The model under review builds one solid part; all positions refer to its coordinate system, in mm. A direction names the side the tool comes from. Round coordinates to 2 decimals unless told otherwise and drop trailing zeros. Order: outer loops, then holes, each group sorted by start corner. A loop starts at its lowest first (then second) coordinate and runs counter-clockwise, first axis right, second up. Notation, with made-up numbers: M 64,87 L 100,87 A32 ccw 100,123 Z; hole C 11.5,48.25 d7. An arc over 180 degrees is marked long. Use a Markdown table: item, result. Add a question column.
1. Insertion check: P1, Ø0.6, axis at x = 4, y = -3, coming from the -Z side; P2, Ø1, axis at y = -2.5, z = 0, coming from the +X side; P3, Ø1, axis at y = -3.5, z = -0.5, coming from the -X side. Each pin has a flat end and moves straight along its axis. Give the tip position at first contact, or say it passes through.
2. Consider section A-A on x = 0. State the section outline as (y, z) points (3 decimals), then the cut area to 3 significant figures.
3. Consider section C-C on y = 12.5. State the section outline as (x, z) points (3 decimals).
4. For faces 1 (the flat face through (-4.6, -2, 0)), 2 (the conical face through (0.734, 20.797, -1.151)), 3 (the flat face through (-0.375, -2, 0)), 4 (the flat face through (-3, 9, -1)), list the 3-axis set-ups (+Z, -Z, +X, -X, +Y, -Y) from which the entire face can be reached by the end or side of a thin tool; tool diameter is ignored.
5. Consider section D-D on x = -5.5. State the section outline as (y, z) points.
6. Consider section B-B on z = 0. State the section outline as (x, y) points (3 decimals).
7. To check wall thickness, follow probe 1 along Y at (x, z) = (-4, 2.75); probe 2 along Y at (x, z) = (2.25, -1); probe 3 along X at (y, z) = (14, -1.5). State the ranges of each line that lie inside material, in increasing order.
from build123d import *

# Parameters (mm, degrees)
SKETCH1_W           = 12.3
SKETCH1_H           = 6.8
BOSS_EXTRUDE1_DEPTH = 9
SKETCH2_R           = 2.925
BOSS_EXTRUDE2_DEPTH = 8.75
SKETCH4_W           = 0.75
SKETCH4_H           = 1.9
BOSS_EXTRUDE3_DEPTH = 4.6


with BuildPart() as part:
    # Sketch1 → Boss-Extrude1 (new body)
    with BuildSketch(Plane(origin=(0, 0, 0), x_dir=(1, 0, 0), z_dir=(0, 1, 0))):
        Rectangle(SKETCH1_W, SKETCH1_H)
    extrude(amount=BOSS_EXTRUDE1_DEPTH)

    # Sketch2 → Boss-Extrude2 (add)
    with BuildSketch(Plane(origin=(0, 9, 0), x_dir=(1, 0, 0), z_dir=(0, 1, 0))):
        Circle(SKETCH2_R)
    extrude(amount=BOSS_EXTRUDE2_DEPTH)

    # Sketch3 → Revolve1 (revolve)
    with BuildSketch(Plane.XY):
        with BuildLine():
            Line((0, 17.75), (1.2, 17.75))
            Line((1.2, 17.75), (1.2, 20.45))
            Line((1.2, 20.45), (2.15, 22.45))
            Line((2.15, 22.45), (1.5, 28.893698303))
            ThreePointArc((1.5, 28.893698303), (1.011132322, 29.860648085), (0, 30.25))
            Line((0, 30.25), (0, 17.75))
        make_face()
    revolve(axis=Axis((0, -982.25, 0), (0, 1, 0)))

    # Sketch4 → Boss-Extrude3 (add)
    with BuildSketch(Plane.XZ):
        Rectangle(SKETCH4_W, SKETCH4_H)
        with Locations((-4.225, 0)):
            Rectangle(SKETCH4_W, SKETCH4_H)
        with Locations((4.225, 0)):
            Rectangle(SKETCH4_W, SKETCH4_H)
    extrude(amount=BOSS_EXTRUDE3_DEPTH)


solid = part.part
Answer block:
| question | item | result |
|---|---|---|
| 1 | P1 | z = -0.95 |
| 1 | P2 | x = 4.6 |
| 1 | P3 | x = -4.6 |
| 2 | outline | M -4.6,-0.95 L 0,-0.95 L 0,-3.4 L 9,-3.4 L 9,-2.925 L 17.75,-2.925 L 17.75,-1.2 L 20.45,-1.2 L 22.45,-2.15 L 28.894,-1.5 A1.508 ccw 28.894,1.5 L 22.45,2.15 L 20.45,1.2 L 17.75,1.2 L 17.75,2.925 L 9,2.925 L 9,3.4 L 0,3.4 L 0,0.95 L -4.6,0.95 Z |
| 2 | area | 161 mm^2 |
| 3 | outline | C 0,0 d5.85 |
| 4 | face 1 | +Z, -Z, -X, -Y |
| 4 | face 2 | none |
| 4 | face 3 | +Z, -Z, -Y |
| 4 | face 4 | +Y |
| 5 | outline | M 0,-3.4 L 9,-3.4 L 9,3.4 L 0,3.4 Z |
| 6 | outline | M -6.15,0 L -4.6,0 L -4.6,-4.6 L -3.85,-4.6 L -3.85,0 L -0.375,0 L -0.375,-4.6 L 0.375,-4.6 L 0.375,0 L 3.85,0 L 3.85,-4.6 L 4.6,-4.6 L 4.6,0 L 6.15,0 L 6.15,9 L 2.925,9 L 2.925,17.75 L 1.2,17.75 L 1.2,20.45 L 2.15,22.45 L 1.5,28.894 A1.508 ccw -1.5,28.894 L -2.15,22.45 L -1.2,20.45 L -1.2,17.75 L -2.925,17.75 L -2.925,9 L -6.15,9 Z |
| 7 | probe 1 | 0 to 9 |
| 7 | probe 2 | 0 to 17.75 |
| 7 | probe 3 | -2.51 to 2.51 |
